Geometry: final body of the model. Coordinates: model frame, mm. Give positions to 0.01 mm unless a question says otherwise; leave off trailing zeros. Order: outer loops, then holes, each group sorted by start corner. A loop starts at its lowest first (then second) coordinate and runs counter-clockwise, first axis right, second up. Notation, with made-up numbers: (-26.75, 64) -> (18.25, 64) arc R14 ccw to (18.25, 89) -> close; hole circle Ø7 at (46.25, -14). An arc over 180 degrees is marked (long way). One line per question, with ' | ' between items. Start each with the question number.
(1) Ray query, L1, parallel to X at y = 0, z = 2.6; L2, parallel to Y at x = -71.12, z = 2.75; L3, parallel to X at y = 0.25, z = 2.6. Return the intervals inside material, ascending.
(2) Section A-A (z = 2.7). Return loops of the section in (x, y).
(3) Section B-B (x = -71.12). Return loops of the section in (y, z), then the cut area to 3 significant figures.
(4) Section C-C (x = -50.8). Return loops of the section in (y, z), then the cut area to 3 significant figures.
(5) Mould query, pull axis X, two halves, no side actions, for faces 1 (the face through (-50.829, -3.698, 2.419)), 2 (the face through (-70, -5.918, 2)), 3 (the face through (5.918, 0, 2)), 4 (the face through (-69.82, 0.06, 2.42)). Classes: +X half, -X half, draft (parallel to the pull), parting line (faces both ways), or undercut.
```python
from build123d import *

# Parameters (mm, degrees)
SKETCH1_W                  = 93.116399905
SKETCH1_H                  = 11.836399908
BOSS_EXTRUDE1_DEPTH        = 1.6002
F_2_6_2_6_DIAMETER_HOLE1_D = 2.6
SKETCH6_W                  = 2.6
SKETCH6_H                  = 0.920741122
CUT_EXTRUDE1_DEPTH         = 2.6002


with BuildPart() as part:
    # Sketch1 → Boss-Extrude1 (new body)
    with BuildSketch(Plane.XY.offset(1.63)):
        with Locations((-40.639999999, 0)):
            Rectangle(SKETCH1_W, SKETCH1_H)
    extrude(amount=BOSS_EXTRUDE1_DEPTH)

    # Ø2.6 (2.6) Diameter Hole1 (through all)
    with Locations(Plane.XY.offset(3.2302)):
        with Locations((-50.800000064, 4.997458832), (-50.800000064, -4.997458832), (-10.160000092, -7.6e-08), (-71.119999812, -3.5e-08)):
            Hole(F_2_6_2_6_DIAMETER_HOLE1_D / 2)

    # Sketch6 → Cut-Extrude1 (cut, through all)
    with BuildSketch(Plane.XY.offset(3.2302)):
        with Locations((-50.800000064, 5.457829393)):
            Rectangle(SKETCH6_W, SKETCH6_H)
        with Locations((-50.800000064, -5.457829393)):
            Rectangle(SKETCH6_W, SKETCH6_H)
    extrude(amount=-CUT_EXTRUDE1_DEPTH, mode=Mode.SUBTRACT)


solid = part.part
```
Response:
1) L1: x = -87.2 to -72.42, -69.82 to -11.46, -8.86 to 5.92 | L2: y = -5.92 to -1.3, 1.3 to 5.92 | L3: x = -87.2 to -72.4, -69.84 to -11.44, -8.88 to 5.92
2) outline: (-87.2, -5.92) -> (-52.1, -5.92) -> (-52.1, -5) arc R1.3 cw to (-49.5, -5) -> (-49.5, -5.92) -> (5.92, -5.92) -> (5.92, 5.92) -> (-49.5, 5.92) -> (-49.5, 5) arc R1.3 cw to (-52.1, 5) -> (-52.1, 5.92) -> (-87.2, 5.92) -> close; hole circle Ø2.6 at (-71.12, 0); hole circle Ø2.6 at (-10.16, 0)
3) outline: (-5.92, 1.63) -> (-1.3, 1.63) -> (-1.3, 3.23) -> (-5.92, 3.23) -> close; (1.3, 1.63) -> (5.92, 1.63) -> (5.92, 3.23) -> (1.3, 3.23) -> close | area: 14.8 mm^2
4) outline: (-3.7, 1.63) -> (3.7, 1.63) -> (3.7, 3.23) -> (-3.7, 3.23) -> close | area: 11.8 mm^2
5) face 1: undercut | face 2: draft | face 3: +X half | face 4: undercut
